Geometry: see drawing. Coordinates: mm, zero at the bounding-box minimum. Give positions to 0.01 mm unless a question says otherwise; leave off trailing zeros. Loops run counter-clockwise (first coordinate to the right, second up) from the corner with the lowest first, then second, coordinate; pieces in that order, holes last. Notation, with made-up numbers: M 71,63.25 L 75,63.25 A37 ccw 75,100.25 Z; hole C -2.5,47 d2. An arc over 180 degrees is marked long. Put each result on its own line as item: value.
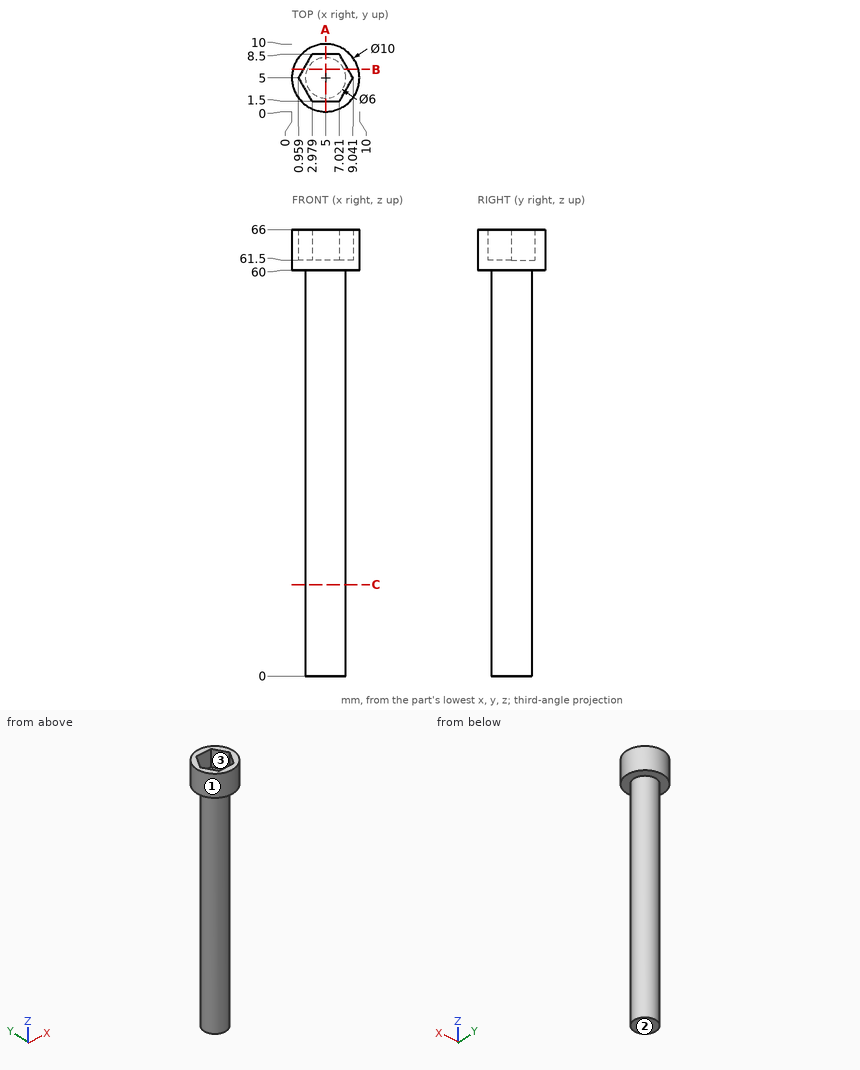
1. Section query C-C (z = 13.5). Output: boundary loops of the cut face in (x, y), plus the area to 3 significant figures.
Found:
outline: C 5,5 d6
area: 28.3 mm^2
2. Section query A-A (x = 5). Output: boundary loops of the cut face in (y, z).
Found:
outline: M 0,60 L 2,60 L 2,0 L 8,0 L 8,60 L 10,60 L 10,66 L 8.5,66 L 8.5,61.5 L 1.5,61.5 L 1.5,66 L 0,66 Z
3. Material intervals for line 1 (Z direction, x = 9.25, y = 2.5); line 2 (Z direction, x = 6.25, y = 6); line 3 (X direction, y = 5.25, z = 19), sorted ascending. Write a range as from..to.
Found:
line 1: 60..66
line 2: 0..61.5
line 3: 2.01..7.99
4. Contact query for flat-ended pins moving along their axis: P1, Ø2, axis at x = 5.5, y = 5, coming from the +Z side; P2, Ø4, axis at y = 1.5, z = 21.5, coming from the +X side; P3, Ø3, axis at x = 6, z = 52.5, coming from the +Y side. Output: stop coordinate, or through.
Found:
P1: z = 61.5
P2: x = 7.6
P3: y = 8
5. Draft query along Y for the marked faces 1, 2 and 3. Return one class per face: pulls with the +Y half, pulls with the -Y half, needs draft (parallel to the pull), parting line crosses it, or undercut.
Found:
face 1: parting line crosses it
face 2: needs draft
face 3: undercut
6. Section query B-B (y = 6.25). Output: boundary loops of the cut face in (x, z).
Found:
outline: M 0.16,60 L 2.27,60 L 2.27,0 L 7.73,0 L 7.73,60 L 9.84,60 L 9.84,66 L 8.32,66 L 8.32,61.5 L 1.68,61.5 L 1.68,66 L 0.16,66 Z
